Can you work these out from the model? Positions are in its coordinate system, mm. Face numbers are marked on the shaded views. A direction names the side the tool comes from. Round coordinates to 2 decimals unless told otherwise and drop trailing zeros. Order: outer loops, then holes, each group sorted by start corner. A loop starts at its lowest first (then second) coordinate and runs counter-clockwise, first axis right, second up. Notation, with made-up numbers: (45, -36) -> (78, -36) arc R30 cw to (78, -10) -> close; hole circle Ø10 at (57.5, 12.5). An arc over 180 degrees is marked (long way). One line per item, written item: value.
```python
from build123d import *

# Parameters (mm, degrees)
SKETCH1_R               = 10.25
BOSS_EXTRUDE1_DEPTH     = 5
SKETCH2_R               = 10.25
BOSS_EXTRUDE2_DEPTH     = 4
CUT_EXTRUDE1_DEPTH      = 18.062385531
CUT_EXTRUDE1_DEPTH_BACK = 2.5
CUT_EXTRUDE2_DEPTH      = 16.333786225
CUT_EXTRUDE2_DEPTH_BACK = 16.333786225
SKETCH4_R               = 1.6
CUT_EXTRUDE3_DEPTH      = 16.333786225
CUT_EXTRUDE3_DEPTH_BACK = 16.333786225
SKETCH5_R               = 2.5


with BuildPart() as part:
    # Sketch1 → Boss-Extrude1 (new body)
    with BuildSketch(Plane.XY):
        Circle(SKETCH1_R)
        Polygon((4.75, 8.227241336), (-4.75, 8.227241336), (-9.5, 0), (-4.75, -8.227241336), (4.75, -8.227241336), (9.5, 0), align=None, mode=Mode.SUBTRACT)
    extrude(amount=BOSS_EXTRUDE1_DEPTH)

    # Sketch2 → Boss-Extrude2 (add)
    with BuildSketch(Plane.XY.offset(5)):
        Circle(SKETCH2_R)
    extrude(amount=BOSS_EXTRUDE2_DEPTH)

    # Sketch3 → Cut-Extrude1 (cut, two sides: drawn at the far end of the back side and taken through both)
    with BuildSketch(Plane.XY.offset(9).offset(-CUT_EXTRUDE1_DEPTH_BACK)):
        with BuildLine():
            ThreePointArc((-3.491027293, 5.482948882), (-6.202138006, 1.94511803), (-5.996942005, -2.507326583))
            Line((-5.996942005, -2.507326583), (-6.770608941, -7.695541213))
            ThreePointArc((-6.770608941, -7.695541213), (-3.067301509, -9.780294548), (1.163287858, -10.183774416))
            Line((1.163287858, -10.183774416), (3.491027293, -5.482948882))
            ThreePointArc((3.491027293, -5.482948882), (6.202138006, -1.94511803), (5.996942005, 2.507326583))
            Line((5.996942005, 2.507326583), (6.770608941, 7.695541213))
            ThreePointArc((6.770608941, 7.695541213), (6.548360484, 7.885523126), (6.32078374, 8.069088728))
            ThreePointArc((6.32078374, 8.069088728), (2.787097923, 9.86380176), (-1.163287858, 10.183774416))
            Line((-1.163287858, 10.183774416), (-3.491027293, 5.482948882))
        make_face()
    extrude(amount=CUT_EXTRUDE1_DEPTH + CUT_EXTRUDE1_DEPTH_BACK, mode=Mode.SUBTRACT)

    # Sketch4 → Cut-Extrude2 (cut, two sides: drawn at the far end of the back side and taken through both)
    with BuildSketch(Plane(origin=(0, 0, 5), x_dir=(-1, 0, 0), z_dir=(0, 0, -1)).offset(-CUT_EXTRUDE2_DEPTH_BACK)):
        with Locations(Location((2.5, -4.330127019, 0), (0, 0, 180))):
            Circle(SKETCH4_R)
        with Locations(Location((-2.5, 4.330127019, 0), (0, 0, 180))):
            Circle(SKETCH4_R)
    extrude(amount=CUT_EXTRUDE2_DEPTH + CUT_EXTRUDE2_DEPTH_BACK, mode=Mode.SUBTRACT)

    # Sketch5 → Cut-Extrude3 (cut, two sides: drawn at the far end of the back side and taken through both)
    with BuildSketch(Plane(origin=(0, 0, 5), x_dir=(-1, 0, 0), z_dir=(0, 0, -1)).offset(-CUT_EXTRUDE3_DEPTH_BACK)):
        with Locations(Location((0, 0, 0), (0, 0, 180))):
            Circle(SKETCH5_R)
    extrude(amount=CUT_EXTRUDE3_DEPTH + CUT_EXTRUDE3_DEPTH_BACK, mode=Mode.SUBTRACT)


solid = part.part
```
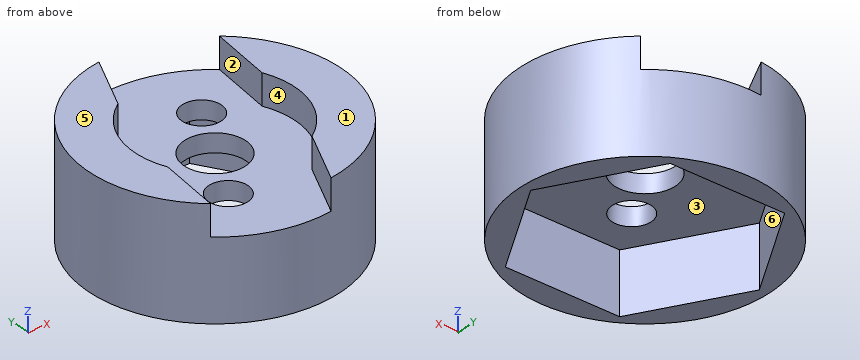
Q1. I want a section at C-C on y = 1. List the corners of the cut face in (x, z) for me, plus the area to 3 significant figures.
Answers below:
outline: (-10.2, 0) -> (-8.92, 0) -> (-8.92, 5) -> (-2.29, 5) -> (-2.29, 6.5) -> (-6.42, 6.5) -> (-6.42, 9) -> (-10.2, 9) -> close; (2.29, 5) -> (8.92, 5) -> (8.92, 0) -> (10.2, 0) -> (10.2, 9) -> (6.42, 9) -> (6.42, 6.5) -> (2.29, 6.5) -> close
area: 55.4 mm^2
Q2. I want a section at A-A on x = 0. List the corners of the cut face in (y, z) for me, plus the area to 3 significant figures.
Answers below:
outline: (-10.25, 0) -> (-8.23, 0) -> (-8.23, 5) -> (-2.5, 5) -> (-2.5, 6.5) -> (-10.25, 6.5) -> close; (2.5, 5) -> (8.23, 5) -> (8.23, 0) -> (10.25, 0) -> (10.25, 6.5) -> (2.5, 6.5) -> close
area: 43.5 mm^2
Q3. I want a section at D-D on z = 3.5. List the corners of the cut face in (x, y) for me, plus the area to 3 significant figures.
Answers below:
outline: circle Ø20.5 at (0, 0); hole (-9.5, 0) -> (-4.75, -8.23) -> (4.75, -8.23) -> (9.5, 0) -> (4.75, 8.23) -> (-4.75, 8.23) -> close
area: 95.6 mm^2
Q4. Please list where these lines run through material, in increasing order: line 1 along Y through (x, z) = (0.5, 3.75); line 2 along X through (y, z) = (-4.25, 4.25); line 3 along X through (y, z) = (-0.5, 7).
Answers below:
line 1: -10.24 to -8.23, 8.23 to 10.24
line 2: -9.33 to -7.05, 7.05 to 9.33
line 3: -10.24 to -6.48, 6.48 to 10.24
Q5. I want a section at B-B on z = 8. List the corners of the cut face in (x, y) for me.
Answers below:
outline: (-6.77, -7.7) -> (-6, -2.51) arc R6.5 cw to (-3.49, 5.48) -> (-1.16, 10.18) arc R10.25 ccw to start; (1.16, -10.18) arc R10.25 ccw to (6.77, 7.7) -> (6, 2.51) arc R6.5 cw to (3.49, -5.48) -> close
Q6. Will these pins go through, and if not, where does the flat tip stop? pin 1 Ø4 at (x, y) = (-2.5, -4.33) entering from -Z; pin 2 Ø1.5 at (x, z) = (-2, 2) entering from -Y; pin 3 Ø1.5 at (x, z) = (-6.5, 2.5) entering from -Y.
Answers below:
pin 1: z = 5
pin 2: y = -10.17
pin 3: y = -8.49
Q7. We'd pull the mould along Y, two halves only. Please class the marked faces 1, 2 and 3: released by +Y, released by -Y, zero draft, split by the parting line, or undercut.
Answers below:
face 1: zero draft
face 2: released by +Y
face 3: undercut
Q8. On a 3-axis mill with a long thin cutter (end or side, diameter ignored), from which of +Z, -Z, +X, -X, +Y, -Y can I reach the whole of each face in a straight line? I mean the marked faces 4, 5 and 6. Say none if no direction works.
Answers below:
face 4: +Z
face 5: +Z, +X, -X, +Y, -Y
face 6: -Z
